Can you work these out from the model? Positions are in its coordinate system, mm. A direction names the side the tool comes from. Give positions to 0.01 mm unless a question says otherwise; leave off trailing zeros. Order: outer loops, then holes, each group sorted by start corner. A loop starts at its lowest first (then second) coordinate and runs counter-clockwise, first axis right, second up. Notation, with made-up numbers: (-32.5, 83.25) - (8.5, 83.25) arc R26 ccw to (8.5, 101.25) - close; hole circle Ø5 at (72.5, -18.5). An arc over 180 degrees is marked (long way). Answer as a JSON object with one key per item and string values.
```python
from build123d import *


with BuildPart() as part:
    # Szkic1 → Obrót1 (revolve)
    with BuildSketch(Plane(origin=(0, 0, 0), x_dir=(0, 0, -1), z_dir=(1, 0, 0))):
        with BuildLine():
            Line((24.687298198, -1.748229667), (-13.312701802, -1.748229667))
            Line((-13.312701802, -1.748229667), (-15.431171619, -1.748229667))
            Line((-15.431171619, -1.748229667), (-15.431171619, 0.751770333))
            Line((-15.431171619, 0.751770333), (-13.312701802, 0.751770333))
            Line((-13.312701802, 0.751770333), (-13.312701802, 3.251770333))
            ThreePointArc((-13.312701802, 3.251770333), (-2.312701802, 0.814239523), (8.687298198, 3.251770333))
            Line((8.687298198, 3.251770333), (8.687298198, 0.751770333))
            Line((8.687298198, 0.751770333), (24.687298198, 0.751770333))
            Line((24.687298198, 0.751770333), (24.687298198, -1.748229667))
        make_face()
    revolve(axis=Axis((0, -1.748229667, -24.687298198), (0, 0, 1)))


solid = part.part
```
Q1. I'm going to push flat-ended pins straight in: pin 1 Ø4 at (x, y) = (3, -3.5) entering from +Z; pin 2 Ø1 at (x, y) = (-3, -4.5) entering from +Z; pin 3 Ø3 at (y, z) = (-3.5, -16.5) entering from +X; pin 4 Ø4 at (y, z) = (-3, 2) entering from -X. Where does each tip first touch, or does it pass through?
Recorded:
{"pin 1": "stops at z = 15.43", "pin 2": "stops at z = 13.31", "pin 3": "stops at x = 2.49", "pin 4": "stops at x = -2.63"}
Q2. I need wall thicknesses on L1, parallel to Y at x = 0, z = -16.5; L2, parallel to Z at x = -4.5, y = -2.5; L3, parallel to Z at x = 2, y = -6.25. Which ranges of each line are inside material? Lowest first, please.
Recorded:
{"L1": "y = -4.25 to 0.75", "L2": "z = -8.69 to -7.69, 12.32 to 13.31", "L3": "z = -8.69 to -8.53, 13.15 to 13.31"}
Q3. If we section it at B-B, the plane z = -17.5: Please give me the cut outline in (x, y).
Recorded:
{"outline": "circle Ø5 at (0, -1.75)"}
Q4. Which directions (+Z, -Z, +X, -X, +Y, -Y) give clear straight access to the entire face, cutting with the end or side of a thin tool? Please do faces 1 (the face through (0, -2, 15.431)), 2 (the face through (2, 0, -8.687)), 3 (the face through (-0.11, -4.246, 14.357)).
Recorded:
{"face 1": "+Z, +X, -X, +Y, -Y", "face 2": "-Z", "face 3": "+Z"}
Q5. If we section it at A-A, the plane x = 0: Please give me the cut outline in (y, z).
Recorded:
{"outline": "(-6.75, -8.69) - (-4.25, -8.69) - (-4.25, -24.69) - (0.75, -24.69) - (0.75, -8.69) - (3.25, -8.69) arc R26.04 cw to (3.25, 13.31) - (0.75, 13.31) - (0.75, 15.43) - (-4.25, 15.43) - (-4.25, 13.31) - (-6.75, 13.31) arc R26.04 cw to start"}
Q6. If we section it at C-C, the plane z = -8: Please give me the cut outline in (x, y), then the cut area to 3 significant figures.
Recorded:
{"outline": "circle Ø9.38 at (0, -1.75)", "area": "69.2 mm^2"}
